```python
from build123d import *

# Parameters (mm, degrees)
CROQUIS1_W                                           = 10.4
CROQUIS1_H                                           = 20.4
SALIENTE_EXTRUIR1_DEPTH                              = 4
CROQUIS2_W                                           = 25.4
CROQUIS2_H                                           = 35.4
SALIENTE_EXTRUIR2_DEPTH                              = 4
CROQUIS3_W                                           = 15
CROQUIS3_H                                           = 15.4
SALIENTE_EXTRUIR3_DEPTH                              = 16.3
CROQUIS4_W                                           = 7.5
CROQUIS4_H                                           = 4
CORTAR_EXTRUIR1_DEPTH                                = 35.907592297
REFRENTADO_PARA_TORNILLO_CON_CABEZA_PLAN_D           = 3.4
REFRENTADO_PARA_TORNILLO_CON_CABEZA_PLAN_CBORE_D     = 6.5
REFRENTADO_PARA_TORNILLO_CON_CABEZA_PLAN_CBORE_DEPTH = 2


with BuildPart() as part:
    # Croquis1 → Saliente-Extruir1 (new body)
    with BuildSketch(Plane(origin=(0, 0, 0), x_dir=(1, 0, 0), z_dir=(0, 1, 0))):
        Rectangle(CROQUIS1_W, CROQUIS1_H)
    extrude(amount=SALIENTE_EXTRUIR1_DEPTH)

    # Croquis2 → Saliente-Extruir2 (add)
    with BuildSketch(Plane(origin=(0, 0, 0), x_dir=(1, 0, 0), z_dir=(0, 1, 0))):
        Rectangle(CROQUIS2_W, CROQUIS2_H)
    extrude(amount=SALIENTE_EXTRUIR2_DEPTH)

    # Croquis3 → Saliente-Extruir3 (add)
    with BuildSketch(Plane(origin=(0, 4, 0), x_dir=(1, 0, 0), z_dir=(0, 1, 0))):
        with Locations((-5.2, 0)):
            Rectangle(CROQUIS3_W, CROQUIS3_H)
    extrude(amount=SALIENTE_EXTRUIR3_DEPTH)

    # Croquis4 → Cortar-Extruir1 (cut, through all)
    with BuildSketch(Plane.XY.offset(7.7)):
        with Locations((-1.45, 14.3)):
            Rectangle(CROQUIS4_W, CROQUIS4_H)
    extrude(amount=-CORTAR_EXTRUIR1_DEPTH, mode=Mode.SUBTRACT)

    # Refrentado para tornillo con cabeza plana de M32 (through all)
    with Locations(Plane(origin=(0, 4, 0), x_dir=(1, 0, 0), z_dir=(0, 1, 0))):
        with Locations((-5.2, 12.7), (-5.2, -12.7), (5.2, -12.7), (5.2, 12.7)):
            CounterBoreHole(REFRENTADO_PARA_TORNILLO_CON_CABEZA_PLAN_D / 2, REFRENTADO_PARA_TORNILLO_CON_CABEZA_PLAN_CBORE_D / 2, REFRENTADO_PARA_TORNILLO_CON_CABEZA_PLAN_CBORE_DEPTH)


solid = part.part
```
Verification items for the finished model (mm, model axes). A direction names the side the tool comes from. Give positions to 0.01 mm unless a question says otherwise; leave off trailing zeros. Loops run counter-clockwise (first coordinate to the right, second up) from the corner with the lowest first, then second, coordinate; pieces in that order, holes last. Notation, with made-up numbers: M 55,-13.5 L 94,-13.5 A6 cw 94,-4.5 Z; hole C 10,62 d4. An arc over 180 degrees is marked long. Return JSON: item names as keys, results as strings.
1) Section check C-C, the plane y = 3.25. Enter the section's corners in (x, z), and give its area (3 significant figures).
Findings:
{"outline": "M -12.7,-17.7 L 12.7,-17.7 L 12.7,17.7 L -12.7,17.7 Z; hole C -5.2,-12.7 d6.5; hole C -5.2,12.7 d6.5; hole C 5.2,-12.7 d6.5; hole C 5.2,12.7 d6.5", "area": "766 mm2"}
2) Tool access check on faces 1 (the flat face through (0, 2, 17.7)), 2 (the cylindrical face through (-2.198, 3.014, -11.455)), 3 (the flat face through (-5, 12, 7.7)). Record the directions out of +Z, -Z, +X, -X, +Y, -Y that give a thin tool (end or side, any length) a straight path to the whole face; none if there is none.
Findings:
{"face 1": "+Z, +X, -X, +Y, -Y", "face 2": "+Y", "face 3": "+Z, +X, -X, +Y"}
3) Section check D-D, the plane x = 5.2. Enter the section's corners in (y, z), and give its area (3 significant figures).
Findings:
{"outline": "M 0,-17.7 L 4,-17.7 L 4,-15.95 L 2,-15.95 L 2,-14.4 L 0,-14.4 Z; M 0,-11 L 2,-11 L 2,-9.45 L 4,-9.45 L 4,9.45 L 2,9.45 L 2,11 L 0,11 Z; M 0,14.4 L 2,14.4 L 2,15.95 L 4,15.95 L 4,17.7 L 0,17.7 Z", "area": "102 mm2"}
4) Material ranges on L1, parallel to X at y = 1.1, z = 12.7; L2, parallel to X at y = 3.4, z = -12.7; L3, parallel to Z at x = 5.2, y = 2.4, recorded low to high. Write a range as [from, to].
Findings:
{"L1": "x = [-12.7, -6.9], [-3.5, 3.5], [6.9, 12.7]", "L2": "x = [-12.7, -8.45], [-1.95, 1.95], [8.45, 12.7]", "L3": "z = [-17.7, -15.95], [-9.45, 9.45], [15.95, 17.7]"}
5) Gauge pin test, flat ends, axial feed: P1, Ø4, axis at x = 5.2, z = -12.7, coming from the -Y side; P2, Ø12, axis at x = -3, y = 13, coming from the +Z side; P3, Ø5, axis at x = -6.5, z = 13.5, coming from the +Y side; P4, Ø6.5, axis at y = 8, z = 3.5, coming from the +X side. Record the tip position at first contact, or that the pin passes through.
Findings:
{"P1": "stops at y = 0", "P2": "stops at z = 7.7", "P3": "stops at y = 4", "P4": "stops at x = 2.3"}
6) Section check A-A, the plane z = -12.7. Enter the section's corners in (x, y).
Findings:
{"outline": "M -12.7,0 L -6.9,0 L -6.9,2 L -8.45,2 L -8.45,4 L -12.7,4 Z; M -3.5,0 L 3.5,0 L 3.5,2 L 1.95,2 L 1.95,4 L -1.95,4 L -1.95,2 L -3.5,2 Z; M 6.9,0 L 12.7,0 L 12.7,4 L 8.45,4 L 8.45,2 L 6.9,2 Z"}
7) Section check B-B, the plane x = -0.5. Enter the section's corners in (y, z).
Findings:
{"outline": "M 0,-17.7 L 4,-17.7 L 4,-7.7 L 12.3,-7.7 L 12.3,7.7 L 4,7.7 L 4,17.7 L 0,17.7 Z; M 16.3,-7.7 L 20.3,-7.7 L 20.3,7.7 L 16.3,7.7 Z"}
8) Mould release check, pull along Z, two halves, no side actions. Record for faces 4 (the cylindrical face through (-4.83, 0.99, -11.04)), 5 (the cylindrical face through (1.953, 3.014, 12.557)), 6 (the flat face through (-5, 12, -7.7)), 7 (the flat face through (2.3, 8, 0)): released by +Z, released by -Z, zero draft, split by the parting line, or undercut.
Findings:
{"face 4": "undercut", "face 5": "undercut", "face 6": "released by -Z", "face 7": "zero draft"}
